Source: CAD feature listing. Evaluate the final solid. Frame: model axes, mm. A direction names the side the tool comes from. Coordinates: 2 decimals unless noted, no trailing zeros.
```python
from build123d import *

# Parameters (mm, degrees)
SKETCH1_R           = 500
BOSS_EXTRUDE1_DEPTH = 100


with BuildPart() as part:
    # Sketch1 → Boss-Extrude1 (new body)
    with BuildSketch(Plane.XY):
        Circle(SKETCH1_R)
    extrude(amount=BOSS_EXTRUDE1_DEPTH)

    # Sketch2 → Revolve2 (revolve)
    with BuildSketch(Plane(origin=(0, 0, 0), x_dir=(1, 0, 0), z_dir=(0, 1, 0)), mode=Mode.PRIVATE) as revolve2_sk:
        with BuildLine():
            Line((191.001086436, -281.617154631), (91.001086436, -281.617154631))
            Line((91.001086436, -281.617154631), (91.001086436, -100))
            Line((91.001086436, -100), (241.001086436, -100))
            add(Edge.make_bspline(
                [(241.001086436, -100), (365.645053483, -541.844977323), (391.001086436, -1000)],
                knots=[0, 0, 0, 1, 1, 1], degree=2))
            Line((391.001086436, -1000), (291.001086436, -1000))
            add(Edge.make_bspline(
                [(191.001086436, -281.617154631), (305.655000956, -631.798317471), (291.001086436, -1000)],
                knots=[0, 0, 0, 1, 1, 1], degree=2))
        make_face()
    revolve(revolve2_sk.sketch.rotate(Axis((0, 0, -166.849755885), (0, 0, 1)), 180), axis=Axis((0, 0, -166.849755885), (0, 0, 1)))


solid = part.part
```
Q1. Material intervals for line 1 along X through (y, z) = (136, 294.5); line 2 along Y through (x, z) = (-210.5, 517); line 3 along Y through (x, z) = (106, 422.5), sorted ascending.
Solutions:
line 1: x = -257.13 to -139.99, 139.99 to 257.13
line 2: y = -261.76 to -140.45, 140.45 to 261.76
line 3: y = -300.16 to -206.05, 206.05 to 300.16
Q2. Set-up query: faces 4 (the flat face through (-118, -215, 100)), 5 (the cylindrical face through (-86.8, -27.33, 189.54)), 6 (the flat face through (-7, 7, 0)). Return all of +Z, -Z, +X, -X, +Y, -Y with unobstructed straight access to the full face (end or side cutting, diameter ignored); none if empty.
Solutions:
face 4: none
face 5: +Z
face 6: -Z, +X, -X, +Y, -Y
Q3. Pin query (flat end, axial travel): P1, Ø1.5, axis at x = 34, z = 491, coming from the +Y side; P2, Ø10, axis at x = -233.5, z = 258.5, coming from the +Y side; P3, Ø3, axis at x = 177, z = 871, coming from the +Y side. Return the tip coordinate at first contact, or that it passes through.
Solutions:
P1: stops at y = 329.7
P2: stops at y = 166.23
P3: stops at y = 339.16
Q4. Pull-direction query (X, two-part tool) for faces 1 (the flat face through (1.8, -291.5, 1000)), 2 (the cylindrical face through (-499.516, 21.984, 49.3)), 3 (the flat face through (-82, 40, 281.617)); classes: pulls with the +X half, pulls with the -X half, needs draft (parallel to the pull), parting line crosses it, or undercut.
Solutions:
face 1: needs draft
face 2: parting line crosses it
face 3: undercut
